Work out the finished part from the listing and answer in its coordinate system (mm). A direction names the side the tool comes from. Give positions to 0.01 mm unless a question says otherwise; leave off trailing zeros. Order: outer loops, then holes, each group sorted by start corner. A loop starts at its lowest first (then second) coordinate and runs counter-clockwise, first axis right, second up. Notation, with made-up numbers: M 24.5,-9 L 46.5,-9 A20 ccw 46.5,26 Z; hole C -26,-36.75 d7. An arc over 180 degrees is marked long. One line per item, written item: value.
from build123d import *

# Parameters (mm, degrees)
SKETCH_1_W      = 1220
SKETCH_1_H      = 910
EXTRUDE_1_DEPTH = 210
SKETCH_2_W      = 60
SKETCH_2_H      = 730
SKETCH_2_W_2    = 920
SKETCH_2_H_2    = 60
EXTRUDE_2_DEPTH = 60
SKETCH_3_W      = 60
SKETCH_3_H      = 60
EXTRUDE_3_DEPTH = 530
EXTRUDE_4_REACH = 1546.053
SKETCH_4_W      = 60
SKETCH_4_H      = 60
EXTRUDE_5_REACH = 1525.516
SKETCH_5_W      = 60
SKETCH_5_H      = 60
SKETCH_6_W      = 690
SKETCH_6_H      = 60
EXTRUDE_7_DEPTH = 980


with BuildPart() as part:
    # ｽｹｯﾁ1 → ﾎﾞｽ - 押し出し1 (new body)
    with BuildSketch(Plane(origin=(0, 0, 0), x_dir=(1, 0, 0), z_dir=(0, 1, 0))):
        with Locations((610, 455)):
            Rectangle(SKETCH_1_W, SKETCH_1_H)
    extrude(amount=EXTRUDE_1_DEPTH)

    # ｽｹｯﾁ2 → ﾎﾞｽ - 押し出し2 (add)
    with BuildSketch(Plane.XZ):
        with Locations((120, -455)):
            Rectangle(SKETCH_2_W, SKETCH_2_H)
        with Locations((610, -140)):
            Rectangle(SKETCH_2_W_2, SKETCH_2_H_2)
        with Locations((610, -770)):
            Rectangle(SKETCH_2_W_2, SKETCH_2_H_2)
        with Locations((1100, -455)):
            Rectangle(SKETCH_2_W, SKETCH_2_H)
    extrude(amount=EXTRUDE_2_DEPTH)

    # ｽｹｯﾁ3 → ﾎﾞｽ - 押し出し3 (add)
    with BuildSketch(Plane(origin=(0, -60, 0), x_dir=(-1, 0, 0), z_dir=(0, -1, 0))):
        with Locations((-120, 140)):
            Rectangle(SKETCH_3_W, SKETCH_3_H)
        with Locations((-1100, 140)):
            Rectangle(SKETCH_3_W, SKETCH_3_H)
        with Locations((-1100, 770)):
            Rectangle(SKETCH_3_W, SKETCH_3_H)
        with Locations((-120, 770)):
            Rectangle(SKETCH_3_W, SKETCH_3_H)
    extrude(amount=EXTRUDE_3_DEPTH)

    # ｽｹｯﾁ4 → ﾎﾞｽ - 押し出し4 (add, up to next)
    with BuildSketch(Plane(origin=(0, 0, -170), x_dir=(-1, 0, 0), z_dir=(0, 0, -1)), mode=Mode.PRIVATE) as extrude_4_sk1:
        with Locations((-120, -470)):
            Rectangle(SKETCH_4_W, SKETCH_4_H)
    extrude_4_tool1 = extrude(extrude_4_sk1.sketch, amount=EXTRUDE_4_REACH, mode=Mode.PRIVATE) - part.part
    # ｽｹｯﾁ4 → ﾎﾞｽ - 押し出し4 (add, up to next)
    with BuildSketch(Plane(origin=(0, 0, -170), x_dir=(-1, 0, 0), z_dir=(0, 0, -1)), mode=Mode.PRIVATE) as extrude_4_sk2:
        with Locations((-120, -240)):
            Rectangle(SKETCH_4_W, SKETCH_4_H)
    extrude_4_tool2 = extrude(extrude_4_sk2.sketch, amount=EXTRUDE_4_REACH, mode=Mode.PRIVATE) - part.part
    # ｽｹｯﾁ4 → ﾎﾞｽ - 押し出し4 (add, up to next)
    with BuildSketch(Plane(origin=(0, 0, -170), x_dir=(-1, 0, 0), z_dir=(0, 0, -1)), mode=Mode.PRIVATE) as extrude_4_sk3:
        with Locations((-1100, -240)):
            Rectangle(SKETCH_4_W, SKETCH_4_H)
    extrude_4_tool3 = extrude(extrude_4_sk3.sketch, amount=EXTRUDE_4_REACH, mode=Mode.PRIVATE) - part.part
    # ｽｹｯﾁ4 → ﾎﾞｽ - 押し出し4 (add, up to next)
    with BuildSketch(Plane(origin=(0, 0, -170), x_dir=(-1, 0, 0), z_dir=(0, 0, -1)), mode=Mode.PRIVATE) as extrude_4_sk4:
        with Locations((-1100, -470)):
            Rectangle(SKETCH_4_W, SKETCH_4_H)
    extrude_4_tool4 = extrude(extrude_4_sk4.sketch, amount=EXTRUDE_4_REACH, mode=Mode.PRIVATE) - part.part
    add(extrude_4_tool1.solids().sort_by_distance((120, -470, -170))[0])
    add(extrude_4_tool2.solids().sort_by_distance((120, -240, -170))[0])
    add(extrude_4_tool3.solids().sort_by_distance((1100, -240, -170))[0])
    add(extrude_4_tool4.solids().sort_by_distance((1100, -470, -170))[0])

    # ｽｹｯﾁ5 → ﾎﾞｽ - 押し出し5 (add, up to next)
    with BuildSketch(Plane(origin=(150, 0, 0), x_dir=(0, 0, -1), z_dir=(1, 0, 0)), mode=Mode.PRIVATE) as extrude_5_sk1:
        with Locations((770, -470)):
            Rectangle(SKETCH_5_W, SKETCH_5_H)
    extrude_5_tool1 = extrude(extrude_5_sk1.sketch, amount=EXTRUDE_5_REACH, mode=Mode.PRIVATE) - part.part
    # ｽｹｯﾁ5 → ﾎﾞｽ - 押し出し5 (add, up to next)
    with BuildSketch(Plane(origin=(150, 0, 0), x_dir=(0, 0, -1), z_dir=(1, 0, 0)), mode=Mode.PRIVATE) as extrude_5_sk2:
        with Locations((140, -470)):
            Rectangle(SKETCH_5_W, SKETCH_5_H)
    extrude_5_tool2 = extrude(extrude_5_sk2.sketch, amount=EXTRUDE_5_REACH, mode=Mode.PRIVATE) - part.part
    add(extrude_5_tool1.solids().sort_by_distance((150, -470, -770))[0])
    add(extrude_5_tool2.solids().sort_by_distance((150, -470, -140))[0])

    # ｽｹｯﾁ6 → ﾎﾞｽ - 押し出し7 (add)
    with BuildSketch(Plane.ZY.offset(-1070)):
        with Locations((-455, -240)):
            Rectangle(SKETCH_6_W, SKETCH_6_H)
    extrude(amount=EXTRUDE_7_DEPTH)


solid = part.part
(1) Which of the six approach directions +Z, -Z, +X, -X, +Y, -Y give full straight-line access (tool end or side, diameter ignored) to faces 1 (the flat face through (1070, -544, -770)), 2 (the flat face through (120, -544, -740)), 3 (the flat face through (1070, -134, -140))?
Findings:
face 1: +Z, -Z, -Y
face 2: +X, -X, -Y
face 3: +Z, -Z
(2) Section D-D, the plane z = -136 is taken. Give the vertices of the cut face in (x, y), then the cut area to 3 significant figures.
Findings:
outline: M 0,0 L 90,0 L 90,-590 L 150,-590 L 150,-500 L 1070,-500 L 1070,-590 L 1130,-590 L 1130,0 L 1220,0 L 1220,210 L 0,210 Z; hole M 150,-440 L 1070,-440 L 1070,-270 L 150,-270 Z; hole M 150,-210 L 1070,-210 L 1070,-60 L 150,-60 Z
area: 493,000 mm^2
(3) Given P1, Ø18, axis at x = 1106.5, y = -108, coming from the -Z side; P2, Ø8, axis at y = -241, z = -369, coming from the -X side; P3, Ø12, axis at x = 673.5, z = -330.5, coming from the -Y side, each flat-ended and moving along its own axis, determine where each tip first touches the part or whether it passes through.
Findings:
P1: stops at z = -800
P2: stops at x = 90
P3: stops at y = -270
(4) Find the intervals of material crossed by probe 1 along Y at (x, z) = (339, -752); probe 2 along Y at (x, z) = (1026, -336.5); probe 3 along Z at (x, y) = (245.5, -442), in increasing order. Write a range as from..to.
Findings:
probe 1: y = -500..-440, -270..-210, -60..210
probe 2: y = -270..-210, 0..210
probe 3: z = -800..-740, -170..-110
(5) Determine the mould class of faces 4 (the flat face through (604, -30, -110)), 5 (the flat face through (150, -544, -770)), 6 (the flat face through (1100, -30, -90)) for opening direction X: pulls with the +X half, pulls with the -X half, needs draft (parallel to the pull), parting line crosses it, or undercut.
Findings:
face 4: undercut
face 5: undercut
face 6: needs draft
(6) Section C-C, the plane x = 391.5 is taken. Give the vertices of the cut face in (y, z).
Findings:
outline: M -500,-800 L -440,-800 L -440,-740 L -500,-740 Z; M -500,-170 L -440,-170 L -440,-110 L -500,-110 Z; M -270,-800 L -210,-800 L -210,-110 L -270,-110 Z; M -60,-800 L 0,-800 L 0,-910 L 210,-910 L 210,0 L 0,0 L 0,-110 L -60,-110 L -60,-170 L 0,-170 L 0,-740 L -60,-740 Z
(7) Section B-B, the plane y = -138.5 is taken. Give the vertices of the cut face in (x, z), then the cut area to 3 significant figures.
Findings:
outline: M 90,-800 L 150,-800 L 150,-740 L 90,-740 Z; M 90,-170 L 150,-170 L 150,-110 L 90,-110 Z; M 1070,-800 L 1130,-800 L 1130,-740 L 1070,-740 Z; M 1070,-170 L 1130,-170 L 1130,-110 L 1070,-110 Z
area: 14,400 mm^2
(8) Section A-A, the plane z = -524 is taken. Give the vertices of the cut face in (x, y).
Findings:
outline: M 0,0 L 90,0 L 90,-60 L 150,-60 L 150,0 L 1070,0 L 1070,-60 L 1130,-60 L 1130,0 L 1220,0 L 1220,210 L 0,210 Z; M 90,-500 L 150,-500 L 150,-440 L 90,-440 Z; M 90,-270 L 1130,-270 L 1130,-210 L 90,-210 Z; M 1070,-500 L 1130,-500 L 1130,-440 L 1070,-440 Z
